```python
from build123d import *

# Parameters (mm, degrees)
F0_W     = 42
F0_H     = 73
F1_DEPTH = 305
F3_DEPTH = 42
F5_DEPTH = 53


with BuildPart() as f1:
    # F0 (on Front) → F1 (new body)
    with BuildSketch(Plane.XZ):
        with Locations((21, 36.5)):
            Rectangle(F0_W, F0_H)
    extrude(amount=-F1_DEPTH)

    # F2 (on face) → F3 (cut)
    with BuildSketch(Plane.YZ.offset(42)):
        Polygon((0, 73), (305, 19), (305, 73), align=None)
    extrude(amount=-F3_DEPTH, mode=Mode.SUBTRACT)

    # F4 (on face) → F5 (cut)
    with BuildSketch(Plane.XZ):
        with BuildLine():
            ThreePointArc((31, 31.2498826658), (31.0000000005, 31.2499413329), (31.0000000007, 31.25))
            ThreePointArc((31.0000000007, 31.25), (28.1442994854, 38.1442827484), (21.2500236693, 41))
            ThreePointArc((21.2500236693, 41), (14.3557172523, 38.1442994847), (11.5000000007, 31.25))
            ThreePointArc((11.5000000007, 31.25), (14.3557088841, 24.3557088834), (21.2500000007, 21.5))
            ThreePointArc((21.2500000007, 21.5), (28.1442496332, 24.3556673997), (31, 31.2498826658))
        make_face()
    extrude(amount=-F5_DEPTH, mode=Mode.SUBTRACT)


solid = f1.part
```
Input: part model. Units: mm. Frame: model coordinates. Give positions to 0.01 mm unless a question says otherwise; leave off trailing zeros. Loops run counter-clockwise (first coordinate to the right, second up) from the corner with the lowest first, then second, coordinate; pieces in that order, holes last. Notation, with made-up numbers: (-0.5, 19) -> (11.5, 19) arc R15 ccw to (11.5, 43) -> close; hole circle Ø3 at (35.25, 78.5). An arc over 180 degrees is marked (long way). Use a Markdown table: item, result.
Q1. Pull-direction query (Z, two-part tool) for faces 1 (the flat face through (21, 150, 0)), 2 (the flat face through (21, 53, 31)), 3 (the flat face through (21, 0, 45)), 4 (the flat face through (21.294, 150.365, 46.378)); classes: pulls with the +Z half, pulls with the -Z half, needs draft (parallel to the pull), parting line crosses it, or undercut.
Entries:
| item | result |
|---|---|
| face 1 | pulls with the -Z half |
| face 2 | undercut |
| face 3 | needs draft |
| face 4 | pulls with the +Z half |
Q2. First-contact query: P1, Ø1.5, axis at x = 28, y = 154.5, coming from the +Z side; P2, Ø10, axis at x = 17.5, z = 31, coming from the -Y side; P3, Ø2, axis at x = 5, y = 234.5, coming from the +Z side. Flat tips, straight axial feed; report the tip coordinate or a pass-through.
Entries:
| item | result |
|---|---|
| P1 | stops at z = 45.78 |
| P2 | stops at y = 53 |
| P3 | stops at z = 31.66 |
Q3. Section query A-A, the plane z = 37. Return the cut outline in (x, y).
Entries:
| item | result |
|---|---|
| outline | (0, 0) -> (13.38, 0) -> (13.38, 53) -> (29.12, 53) -> (29.12, 0) -> (42, 0) -> (42, 203.33) -> (0, 203.33) -> close |
Q4. Ray query, probe 1 along Z at (x, y) = (33, 113); probe 2 along Z at (x, y) = (11, 176.5); probe 3 along Z at (x, y) = (23, 17.5). Return the intervals inside material, ascending. Write a range as from..to.
Entries:
| item | result |
|---|---|
| probe 1 | z = 0..52.99 |
| probe 2 | z = 0..41.75 |
| probe 3 | z = 0..21.66, 40.84..69.9 |
Q5. Section query D-D, the plane y = 247. Return the cut outline in (x, z).
Entries:
| item | result |
|---|---|
| outline | (0, 0) -> (42, 0) -> (42, 29.27) -> (0, 29.27) -> close |
Q6. Section query B-B, the plane x = 14.5. Return the cut outline in (y, z), plus the area to 3 significant figures.
Entries:
| item | result |
|---|---|
| outline | (0, 0) -> (305, 0) -> (305, 19) -> (0, 73) -> (0, 38.29) -> (53, 38.29) -> (53, 24.21) -> (0, 24.21) -> close |
| area | 13,300 mm² |
